Design review of the part built by this model. Coordinates are the model's own, in mm. Coordinates: 2 decimals unless noted, no trailing zeros. Loops run counter-clockwise (first coordinate to the right, second up) from the corner with the lowest first, then second, coordinate; pieces in that order, holes last. Notation, with made-up numbers: M -16,56 L 10,56 A10 ccw 10,74 Z; hole C 73.25,79.25 d2. An arc over 180 degrees is marked long. Put each result on its own line as item: value. Start each with the question number.
(1) Take a section at A-A, the plane z = 0. Give the boundary of the cut face in (x, y) (3 decimals), then the cut area to 3 significant figures.
(2) Clearance check with flat-ended pins moving along their axes: pin 1 (1 mm diameter, centred on y = 1.5, z = 64.5, fed in from -X); pin 2 (1.6 mm diameter, centred on y = 1, z = -32.5, fed in from +X); pin 3 (1 mm diameter, centred on x = 34, y = 2, fed in from -Z). State where each tip first meets the part, or that it passes through.
(3) Take a section at B-B, the plane x = -56. Give the boundary of the cut face in (y, z) (3 decimals).
(4) Take a section at C-C, the plane y = 0.65. Count the separate pieces of the cut face and the enclosed holes in it, then the cut area to 3 significant figures.
(5) Take a section at D-D, the plane z = 83.5. Give the boundary of the cut face in (x, y) (3 decimals), then the cut area to 3 significant figures.
(6) For probe 1 along Z at (x, y) = (-46, 0.65); probe 2 along Z at (x, y) = (-46.5, 1.85); probe 3 along X at (y, z) = (1.3, 37), list the stretches that pass through material, from the lowest coordinate up. Write a range as [from, to].
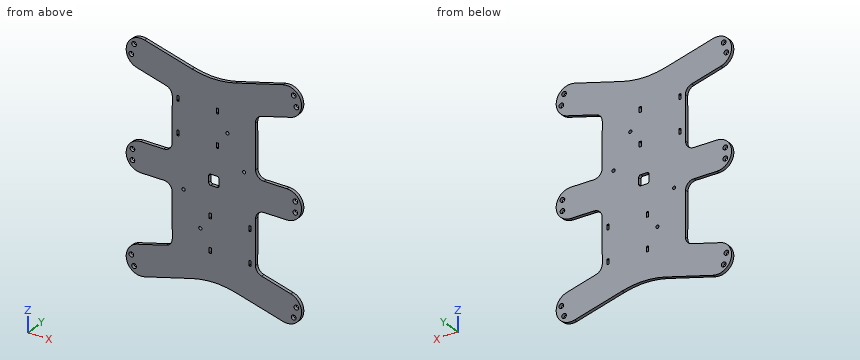
```python
from build123d import *

# Parameters (mm, degrees)
BOSS_EXTRUDE1_DEPTH = 3.175
FILLET1_R           = 80
FILLET2_R           = 8
SKETCH7_R           = 2.25
CUT_EXTRUDE4_DEPTH  = 10
CUT_EXTRUDE5_DEPTH  = 10
SKETCH9_W           = 10
SKETCH9_H           = 10
CUT_EXTRUDE6_DEPTH  = 10
FILLET3_R           = 2
SKETCH12_W          = 2
SKETCH12_H          = 5
CUT_EXTRUDE7_DEPTH  = 10


with BuildPart() as part:
    # Sketch1 → Boss-Extrude1 (new body)
    with BuildSketch(Plane(origin=(0, 0, 0), x_dir=(1, 0, 0), z_dir=(0, 1, 0))):
        with BuildLine():
            Line((-70, 14), (-40, 14))
            Line((-40, 14), (-39.816062711, 70))
            Line((-39.816062711, 70), (-73.623466631, 79.058666579))
            ThreePointArc((-73.623466631, 79.058666579), (-83.522961568, 96.205094778), (-66.376533369, 106.104589715))
            Line((-66.376533369, 106.104589715), (0, 88.319051202))
            Line((0, 88.319051202), (66.376533369, 106.104589715))
            ThreePointArc((66.376533369, 106.104589715), (83.522961568, 96.205094778), (73.623466631, 79.058666579))
            Line((73.623466631, 79.058666579), (39.816062711, 70))
            Line((39.816062711, 70), (40, 14))
            Line((40, 14), (70, 14))
            ThreePointArc((70, 14), (84, 0), (70, -14))
            Line((70, -14), (40, -14))
            Line((40, -14), (39.816062711, -70))
            Line((39.816062711, -70), (73.623466631, -79.058666579))
            ThreePointArc((73.623466631, -79.058666579), (83.522961568, -96.205094778), (66.376533369, -106.104589715))
            Line((66.376533369, -106.104589715), (0, -88.319051202))
            Line((0, -88.319051202), (-66.376533369, -106.104589715))
            ThreePointArc((-66.376533369, -106.104589715), (-83.522961568, -96.205094778), (-73.623466631, -79.058666579))
            Line((-73.623466631, -79.058666579), (-39.816062711, -70))
            Line((-39.816062711, -70), (-40, -14))
            Line((-40, -14), (-70, -14))
            ThreePointArc((-70, -14), (-84, 0), (-70, 14))
        make_face()
    extrude(amount=BOSS_EXTRUDE1_DEPTH)

    # Fillet1
    fillet1_edges = [part.edges().sort_by_distance(p)[0] for p in [
        (0, 1.5875, -88.319051202),
        (0, 1.5875, 88.319051202),
    ]]
    fillet(fillet1_edges, radius=FILLET1_R)

    # Fillet2
    fillet2_edges = [part.edges().sort_by_distance(p)[0] for p in [
        (-40, 1.5875, -14),
        (-39.816062711, 1.5875, -70),
        (39.816062711, 1.5875, -70),
        (40, 1.5875, -14),
        (40, 1.5875, 14),
        (39.816062711, 1.5875, 70),
        (-39.816062711, 1.5875, 70),
        (-40, 1.5875, 14),
    ]]
    fillet(fillet2_edges, radius=FILLET2_R)

    # Sketch7 → Cut-Extrude4 (cut)
    with BuildSketch(Plane(origin=(0, 3.175, 0), x_dir=(1, 0, 0), z_dir=(0, 1, 0))):
        with Locations(Location((-76.433311385, -99.481809639, 0), (0, 0, 270))):
            Circle(SKETCH7_R)
        with Locations(Location((-79.021501836, -89.822551376, 0), (0, 0, 270))):
            Circle(SKETCH7_R)
        with Locations(Location((-78, -5, 0), (0, 0, 270))):
            Circle(SKETCH7_R)
        with Locations(Location((-78, 5, 0), (0, 0, 270))):
            Circle(SKETCH7_R)
        with Locations(Location((-79.021501836, 89.822551376, 0), (0, 0, 270))):
            Circle(SKETCH7_R)
        with Locations(Location((-76.433311385, 99.481809639, 0), (0, 0, 270))):
            Circle(SKETCH7_R)
        with Locations(Location((79.021501836, 89.822551376, 0), (0, 0, 270))):
            Circle(SKETCH7_R)
        with Locations(Location((76.433311385, 99.481809639, 0), (0, 0, 270))):
            Circle(SKETCH7_R)
        with Locations(Location((78, -5, 0), (0, 0, 270))):
            Circle(SKETCH7_R)
        with Locations(Location((78, 5, 0), (0, 0, 270))):
            Circle(SKETCH7_R)
        with Locations(Location((79.021501836, -89.822551376, 0), (0, 0, 270))):
            Circle(SKETCH7_R)
        with Locations(Location((76.433311385, -99.481809639, 0), (0, 0, 270))):
            Circle(SKETCH7_R)
    extrude(amount=-CUT_EXTRUDE4_DEPTH, mode=Mode.SUBTRACT)

    # Sketch8 → Cut-Extrude5 (cut)
    with BuildSketch(Plane(origin=(0, 3.175, 0), x_dir=(1, 0, 0), z_dir=(0, 1, 0))):
        with BuildLine():
            ThreePointArc((13, -45), (11.5, -46.5), (13, -48))
            ThreePointArc((13, -48), (14.5, -46.5), (13, -45))
        make_face()
        with BuildLine():
            ThreePointArc((29, -15), (27.5, -16.5), (29, -18))
            ThreePointArc((29, -18), (30.5, -16.5), (29, -15))
        make_face()
        with BuildLine():
            ThreePointArc((-13, 48), (-14.5, 46.5), (-13, 45))
            ThreePointArc((-13, 45), (-11.5, 46.5), (-13, 48))
        make_face()
        with BuildLine():
            ThreePointArc((-29, 18), (-30.5, 16.5), (-29, 15))
            ThreePointArc((-29, 15), (-27.5, 16.5), (-29, 18))
        make_face()
    extrude(amount=-CUT_EXTRUDE5_DEPTH, mode=Mode.SUBTRACT)

    # Sketch9 → Cut-Extrude6 (cut)
    with BuildSketch(Plane(origin=(0, 3.175, 0), x_dir=(1, 0, 0), z_dir=(0, 1, 0))):
        Rectangle(SKETCH9_W, SKETCH9_H)
    extrude(amount=-CUT_EXTRUDE6_DEPTH, mode=Mode.SUBTRACT)

    # Fillet3
    fillet3_edges = [part.edges().sort_by_distance(p)[0] for p in [
        (-5, 1.5875, 5),
        (-5, 1.5875, -5),
        (5, 1.5875, -5),
        (5, 1.5875, 5),
    ]]
    fillet(fillet3_edges, radius=FILLET3_R)

    # Sketch12 → Cut-Extrude7 (cut)
    with BuildSketch(Plane(origin=(0, 3.175, 0), x_dir=(1, 0, 0), z_dir=(0, 1, 0))):
        with Locations((-34.5, -32.5)):
            Rectangle(SKETCH12_W, SKETCH12_H)
        with Locations((-34.5, -63.5)):
            Rectangle(SKETCH12_W, SKETCH12_H)
        with Locations((3.5, -63.5)):
            Rectangle(SKETCH12_W, SKETCH12_H)
        with Locations((3.5, -32.5)):
            Rectangle(SKETCH12_W, SKETCH12_H)
        with Locations((-3.5, 63.5)):
            Rectangle(SKETCH12_W, SKETCH12_H)
        with Locations((-3.5, 32.5)):
            Rectangle(SKETCH12_W, SKETCH12_H)
        with Locations((34.5, 32.5)):
            Rectangle(SKETCH12_W, SKETCH12_H)
        with Locations((34.5, 63.5)):
            Rectangle(SKETCH12_W, SKETCH12_H)
    extrude(amount=-CUT_EXTRUDE7_DEPTH, mode=Mode.SUBTRACT)


solid = part.part
```
Computed values:
1. outline: M -84,0 L -5,0 L -5,3.175 L -84,3.175 Z; M 5,0 L 84,0 L 84,3.175 L 5,3.175 Z
1. area: 502 mm^2
2. pin 1: stops at x = -39.92
2. pin 2: stops at x = 39.94
2. pin 3: stops at z = -97.56
3. outline: M 0,-103.324 L 3.175,-103.324 L 3.175,-74.336 L 0,-74.336 Z; M 0,-14 L 3.175,-14 L 3.175,14 L 0,14 Z; M 0,74.336 L 3.175,74.336 L 3.175,103.324 L 0,103.324 Z
4. separate pieces: 1
4. enclosed holes: 25
4. area: 21,700 mm^2
5. outline: M -80.655,0 L 80.655,0 L 80.655,3.175 L -80.655,3.175 Z
5. area: 512 mm^2
6. probe 1: z = [-100.64, -71.66], [-14.25, 14.25], [71.66, 100.64]
6. probe 2: z = [-100.78, -71.79], [-14.14, 14.14], [71.79, 100.78]
6. probe 3: x = [-39.92, 39.92]
